The figure shows three views and two pictorial views of one solid part (mm, origin at its lowest corner). Answer the questions. Give positions to 0.01 mm unless a question says otherwise; leave off trailing zeros. Loops run counter-clockwise (first coordinate to the right, second up) from the corner with the lowest first, then second, coordinate; pieces in that order, holes last. Notation, with made-up numbers: (-13, -29.5) - (40, -29.5) arc R21 cw to (40, -14.5) - close; hole circle Ø1 at (17.25, 44). An arc over 180 degrees is marked (long way). One line per question, with ' | ' between items.
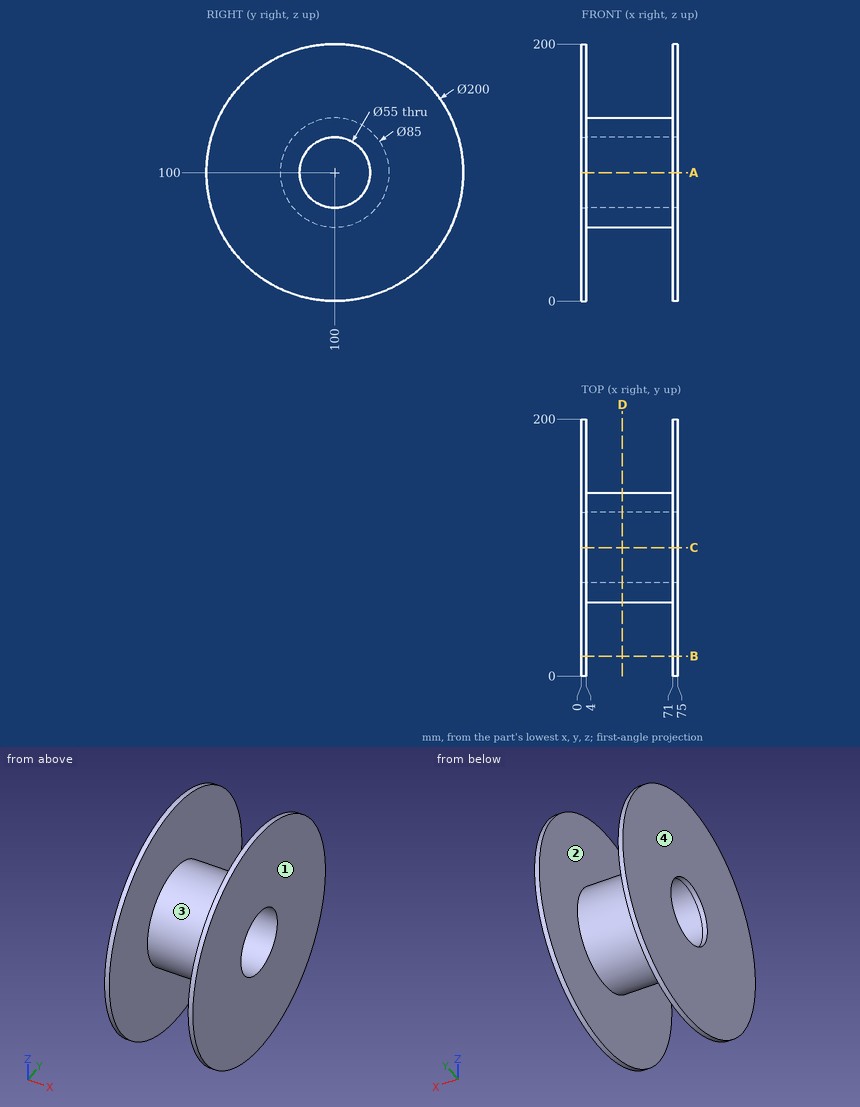
1. Determine the mould class of the marked faces 1, 2, 3 and 4 for opening direction X: +X half, -X half, draft (parallel to the pull), parting line (faces both ways), or undercut.
Evaluation:
face 1: +X half | face 2: undercut | face 3: undercut | face 4: -X half
2. Flat-ended cylindrical pins translate along their axes: pin 1 (6 mm diameter, centred on x = 59.5, z = 93, fed in from +Y); pin 2 (8 mm diameter, centred on x = 65.5, y = 90, fed in from +Z); pin 3 (3 mm diameter, centred on x = 32, z = 124.5, fed in from +Y). Find the tip coordinate at first contact, or state that the pin passes through.
Evaluation:
pin 1: y = 142.31 | pin 2: z = 142.07 | pin 3: y = 135.74
3. Consider L1, parallel to X at y = 143.5, z = 49.5; L2, parallel to Z at x = 23, y = 100; L3, parallel to Z at x = 1, y = 100. Determine where each line is inside the solid, lowest interval first.
Evaluation:
L1: 0 to 4, 71 to 75 | L2: 57.5 to 72.5, 127.5 to 142.5 | L3: 0 to 72.5, 127.5 to 200
4. Find section B-B on y = 15.5. Write down the section's boundary in (x, z).
Evaluation:
outline: (0, 46.52) - (4, 46.52) - (4, 153.48) - (0, 153.48) - close; (71, 46.52) - (75, 46.52) - (75, 153.48) - (71, 153.48) - close
5. Find section D-D on x = 32. Write down the section's boundary in (y, z), then the cut area to 3 significant figures.
Evaluation:
outline: circle Ø85 at (100, 100); hole circle Ø55 at (100, 100) | area: 3,300 mm2
6. Find section A-A on z = 100. Write down the section's boundary in (x, y).
Evaluation:
outline: (0, 0) - (4, 0) - (4, 57.5) - (71, 57.5) - (71, 0) - (75, 0) - (75, 72.5) - (0, 72.5) - close; (0, 127.5) - (75, 127.5) - (75, 200) - (71, 200) - (71, 142.5) - (4, 142.5) - (4, 200) - (0, 200) - close
